Here's how the part is built. I have some questions about the finished solid (model axes, mm). Face numbers are marked on the shaded views. Round coordinates to 2 decimals unless told otherwise and drop trailing zeros. Write each loop counter-clockwise with the first axis right and the second up, starting at its lowest first coordinate (ties: lowest second). Pieces come first, ordered by that corner, then holes. Notation, with made-up numbers: M -15.5,11 L 38.5,11 A19 cw 38.5,38 Z; hole C 22.25,-4.75 d7. An arc over 180 degrees is marked long. Write item = value, one per line. Start each with the question number.
(1) I want a section at A-A (z = 29). List the corners of the cut face in (x, y) for me, and give its area (3 significant figures).
(2) Will this pin go through, and if not, where does the flat tip stop? pin 1 Ø15 at (y, z) = (1, 30.5) entering from -X.
(3) I want a section at B-B (y = 0). List the corners of the cut face in (x, z) for me, and give its area (3 significant figures).
(4) If we mould it in two halves opening along Y, with no side actions, what happens to the marked faces 1, 2 and 3? For each: released by +Y, released by -Y, zero draft, split by the parting line, or undercut.
(5) I need wall thicknesses on line 1 along Z through (x, y) = (13, 0); line 2 along Y through (x, z) = (149.5, 3.5); line 3 along X through (y, z) = (3, 30). Which ranges of each line are inside material? Lowest first, please.
```python
from build123d import *

# Parameters (mm, degrees)
F1_DEPTH = 225
F3_R     = 9.5
F4_DEPTH = 52


with BuildPart() as f1:
    # F0 (on Right) → F1 (new body)
    with BuildSketch(Plane.YZ):
        Polygon((3, 6), (3, 0), (32.5, 0), (32.5, 65), (0, 65), (0, 6), align=None)
    extrude(amount=F1_DEPTH)

    # F2: F1 across plane


with BuildPart() as f1_1:
    add(f1.part)
    add(f1.part.mirror(Plane.XZ))

    # F3 (on Right) → F4 (cut)
    with BuildSketch(Plane.YZ):
        with Locations((0, 29)):
            Circle(F3_R)
    extrude(amount=F4_DEPTH, mode=Mode.SUBTRACT)


solid = f1_1.part
```
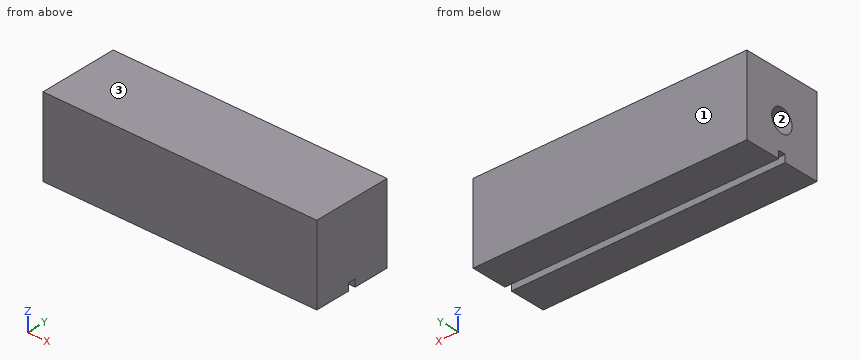
Returned:
q1.outline = M 0,-32.5 L 225,-32.5 L 225,32.5 L 0,32.5 L 0,9.5 L 52,9.5 L 52,-9.5 L 0,-9.5 Z
q1.area = 13,600 mm²
q2.pin_1 = 52
q3.outline = M 0,6 L 225,6 L 225,65 L 0,65 L 0,38.5 L 52,38.5 L 52,19.5 L 0,19.5 Z
q3.area = 12,300 mm²
q4.face_1 = released by +Y
q4.face_2 = undercut
q4.face_3 = zero draft
q5.line_1 = 6 to 19.5, 38.5 to 65
q5.line_2 = -32.5 to -3, 3 to 32.5
q5.line_3 = 52 to 225
